Geometry check sheet. Reference: drawing and pictorial views, mm from the part's lowest x, y, z. Round coordinates to 2 decimals unless told otherwise and drop trailing zeros. Order: outer loops, then holes, each group sorted by start corner. A loop starts at its lowest first (then second) coordinate and runs counter-clockwise, first axis right, second up.
(1) Sectioned sample at A-A, the plane z = 4. Enter the section's corners in (x, y).
(2) Sectioned sample at C-C, the plane z = 27. Enter the section's corners in (x, y).
(3) Mould release check, pull along X, two halves, no side actions. Record for the marked faces 1 and 2: released by +X, released by -X, zero draft, split by the parting line, or undercut.
(4) Sectioned sample at D-D, the plane x = 66. Enter the section's corners in (y, z), and give its area (3 significant figures).
(5) Sectioned sample at B-B, the plane x = 10. Enter the section's corners in (y, z).
(6) Thickness scan on probe 1 along Z at (x, y) = (110, 4.95); probe 2 along Z at (x, y) = (10, 1.05); probe 3 along Y at (x, z) = (77, 41). Record the ranges inside material, lowest first.
(7) Depth check by flat-ended pin: pin 1 (1.7 mm diameter, centred on x = 11.5, z = 4.5, fed in from +Y). Enter the tip coordinate at first touch or a pass-through.
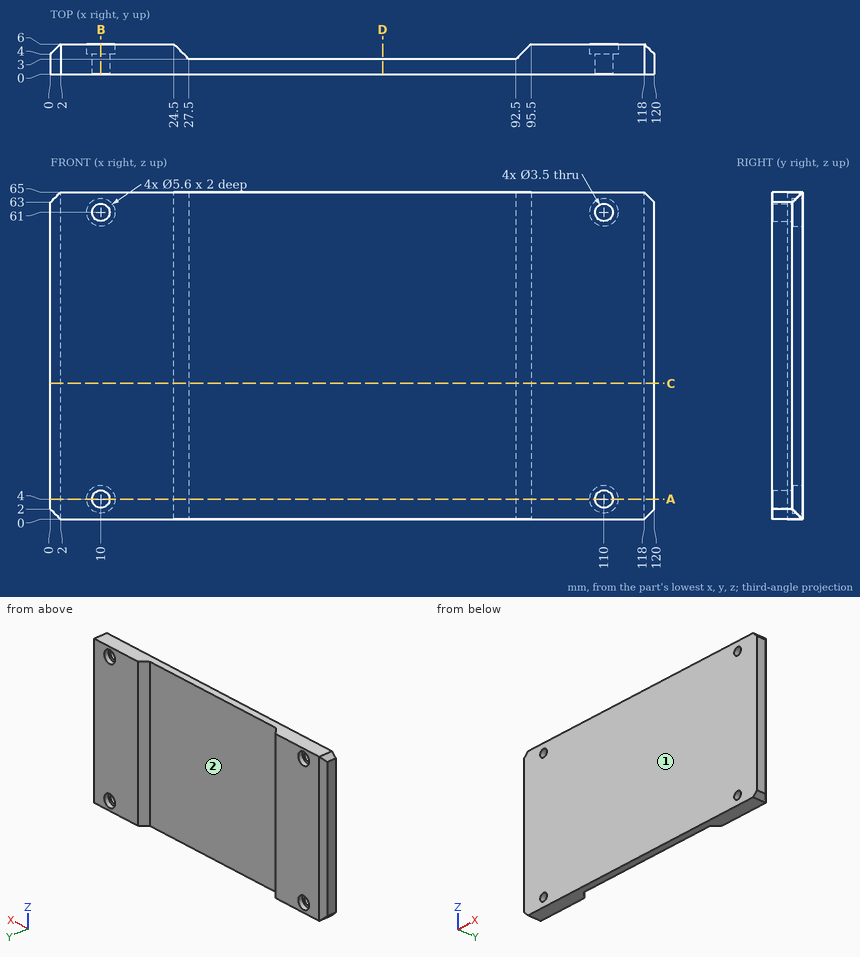
Derived:
1. outline: (0, 0) - (8.25, 0) - (8.25, 4) - (7.2, 4) - (7.2, 6) - (2, 6) - (0, 4) - close; (11.75, 0) - (108.25, 0) - (108.25, 4) - (107.2, 4) - (107.2, 6) - (95.5, 6) - (92.5, 3) - (27.5, 3) - (24.5, 6) - (12.8, 6) - (12.8, 4) - (11.75, 4) - close; (111.75, 0) - (120, 0) - (120, 4) - (118, 6) - (112.8, 6) - (112.8, 4) - (111.75, 4) - close
2. outline: (0, 0) - (120, 0) - (120, 4) - (118, 6) - (95.5, 6) - (92.5, 3) - (27.5, 3) - (24.5, 6) - (2, 6) - (0, 4) - close
3. face 1: zero draft
3. face 2: undercut
4. outline: (0, 0) - (3, 0) - (3, 65) - (0, 65) - close
4. area: 195 mm2
5. outline: (0, 0) - (6, 0) - (6, 1.2) - (4, 1.2) - (4, 2.25) - (0, 2.25) - close; (0, 5.75) - (4, 5.75) - (4, 6.8) - (6, 6.8) - (6, 58.2) - (4, 58.2) - (4, 59.25) - (0, 59.25) - close; (0, 62.75) - (4, 62.75) - (4, 63.8) - (6, 63.8) - (6, 65) - (0, 65) - close
6. probe 1: z = 0 to 1.2, 6.8 to 58.2, 63.8 to 65
6. probe 2: z = 0 to 2.25, 5.75 to 59.25, 62.75 to 65
6. probe 3: y = 0 to 3
7. pin 1: stops at y = 4
